Could you check a few things on this drawing? It's one solid part, dimensions in mm from its lowest x, y, z. Round coordinates to 2 decimals unless told otherwise and drop trailing zeros. Loops run counter-clockwise (first coordinate to the right, second up) from the corner with the lowest first, then second, coordinate; pieces in that order, holes last. Notation, with made-up numbers: M 36,82 L 51,82 A19 cw 51,104 Z; hole C -14.5,33 d6. An arc over 180 degrees is marked long. Write each question's results on one line, items separated by ' | '. Start each with the question number.
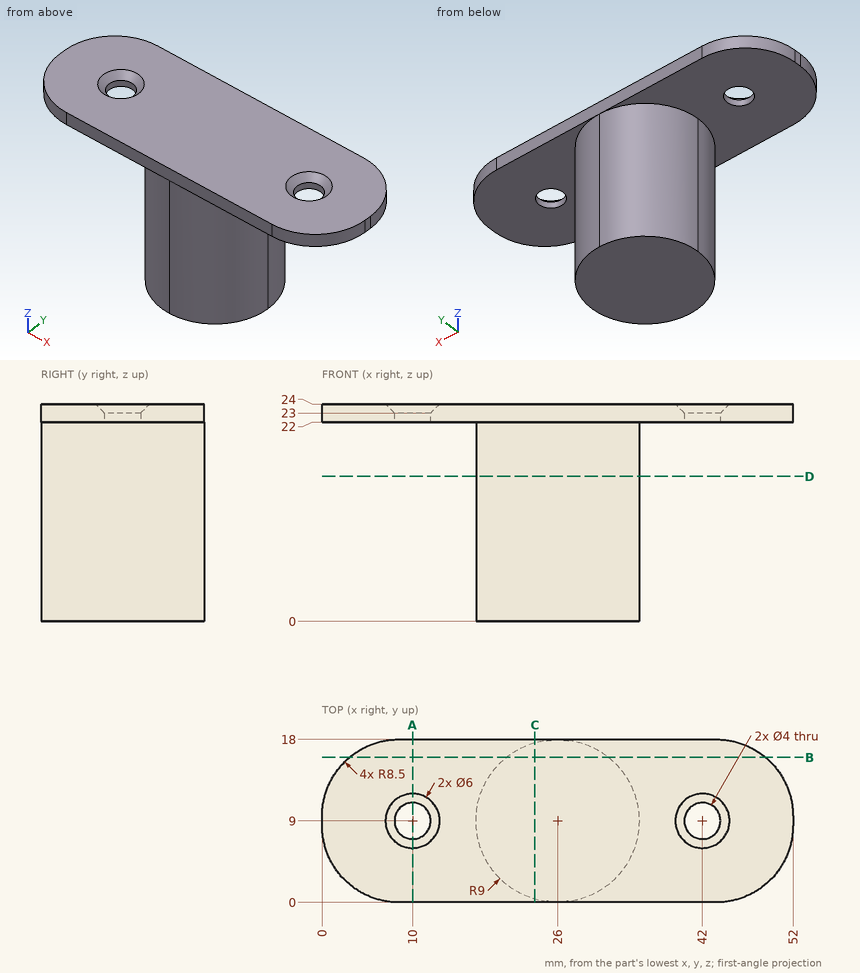
1. I want a section at D-D on z = 16. List the corners of the cut face in (x, y) for me.
2. I want a section at A-A on x = 10. List the corners of the cut face in (y, z) for me, plus the area to 3 significant figures.
3. I want a section at C-C on x = 23.5. List the corners of the cut face in (y, z) for me, plus the area to 3 significant figures.
4. For pin 1 (1 mm diameter, centred on y = 15.5, z = 20, fed in from -X); pin 2 (3 mm diameter, centred on x = 42.5, y = 10, fed in from +Z), each with a flat end and sliding along its axis, tell me the tip position at first contact or that it passes through.
5. I want a section at B-B on y = 16. List the corners of the cut face in (x, z) for me.
6. I need wall thicknesses on line 1 along Y through (x, z) = (10, 22.4); line 2 along Z through (x, y) = (3, 8); line 3 along X through (y, z) = (3, 19). Which ranges of each line are inside material? Lowest first, please.
Outcome:
1) outline: C 26,9 d18
2) outline: M 0,22 L 7,22 L 7,23 L 6,24 L 0,24 Z; M 11,22 L 18,22 L 18,24 L 12,24 L 11,23 Z | area: 27.0 mm2
3) outline: M 0,22 L 0.35,22 L 0.35,0 L 17.65,0 L 17.65,22 L 18,22 L 18,24 L 0,24 Z | area: 416 mm2
4) pin 1: x = 19.29 | pin 2: z = 23.62
5) outline: M 3.02,22 L 20.34,22 L 20.34,0 L 31.66,0 L 31.66,22 L 48.98,22 L 48.98,24 L 3.02,24 Z
6) line 1: 0 to 7, 11 to 18 | line 2: 22 to 24 | line 3: 19.29 to 32.71
